Autodesk Inventor part; units mm, degrees
ref_plane "YZ Plane" through (0, 0, 0) normal (1, 0, 0) x (0, 1, 0)
ref_plane "XZ Plane" through (0, 0, 0) normal (0, 1, 0) x (-1, 0, 0)
ref_plane "XY Plane" through (0, 0, 0) normal (0, 0, 1) x (1, 0, 0)
sketch "Sketch1" plane through (0, 0, 0) normal (0, 0, 1) x (1, 0, 0)
  circle A0 centre (15.5, -7) radius 1.6
  circle A1 centre (7.75, -20.4234) radius 1.6
  circle A2 centre (-7.75, -20.4234) radius 1.6
  circle A3 centre (-15.5, -7) radius 1.6
  circle A4 centre (7.75, 6.4234) radius 1.6
  circle A5 centre (-7.75, 6.4234) radius 1.6
  circle A6 centre (0, 0) radius 6
  arc A7 (20, -7) -> (-20, -7) centre (0, -7) ccw
  line L0 (20, -7) -> (20, -32)
  line L1 (20, -32) -> (-20, -32)
  line L2 (-20, -32) -> (-20, -7)
  dimension "d0" = 40
  dimension "d1" = 25
extrude "Extrusion1" add sketch "Sketch1" along normal blind 3
sketch "Sketch2" plane through (-20, -32, 0) normal (0, -1, 0) x (1, 0, 0)
  line L0 (0, 0) -> (0, 3)
  line L1 (0, 3) -> (40, 3)
  line L2 (40, 3) -> (40, -70)
  line L3 (40, -70) -> (0, -70)
  line L4 (0, -70) -> (0, 3)
  line L5 (0, -70) -> (40, -70)
  line L6 (40, -70) -> (40, -25)
  line L7 (40, -25) -> (0, -25) construction
  line L8 (0, -25) -> (0, -70)
  line L9 (40, -25) -> (0, -70) construction
  line L10 (36.5, -30) -> (3.5, -30) construction
  line L11 (3.5, -30) -> (3.5, -65) construction
  line L12 (3.5, -65) -> (36.5, -65) construction
  line L13 (36.5, -65) -> (36.5, -30) construction
  line L14 (36.5, -30) -> (3.5, -65) construction
  line L15 (3.5, -30) -> (36.5, -65) construction
  circle A0 centre (36.5, -30) radius 1.55
  circle A1 centre (36.5, -65) radius 1.55
  circle A2 centre (3.5, -30) radius 1.55
  circle A3 centre (3.5, -65) radius 1.55
  point P0 (20, 0)
  point P1 (20, -47.5)
  dimension "d4" = 73
  dimension "d5" = 45
  dimension "d6" = 33
  dimension "d7" = 35
  dimension "d8" = 3.1
  dimension "d11" = 35
  dimension "d14" = 33
extrude "Extrusion2" add sketch "Sketch2" against normal blind 3
properties part number "Push_motor_fix"
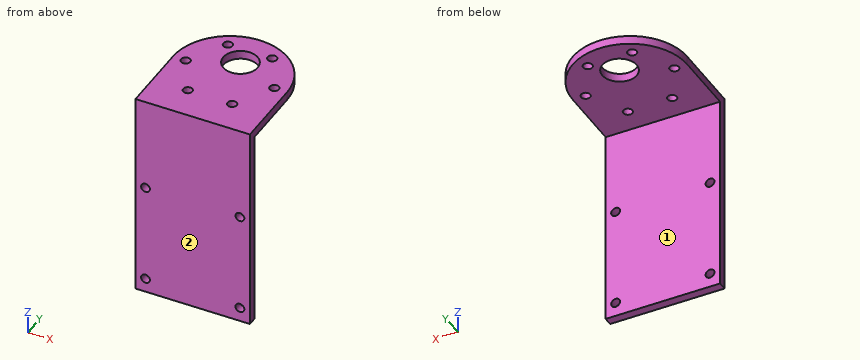
Input: part model. Units: mm. Frame: model coordinates. Face numbers are marked on the shaded views. A direction names the side the tool comes from. Coordinates: 2 decimals unless noted, no trailing zeros. Loops run counter-clockwise (first coordinate to the right, second up) from the corner with the lowest first, then second, coordinate; pieces in that order, holes last. Notation, with made-up numbers: (41, 39) -> (70, 39) arc R18 ccw to (70, 48) -> close; hole circle Ø3 at (-40, 25). An arc over 180 degrees is marked (long way). One line per item, written item: value.
(1) Pin query (flat end, axial travel): pin 1 Ø20 at (x, z) = (5, -20) entering from +Y; pin 2 Ø4 at (x, y) = (-15.5, -7) entering from -Z. Return the tip coordinate at first contact, or that it passes through.
Answer below:
pin 1: stops at y = -29
pin 2: stops at z = 0
(2) Cut plane D-D (x = -7.75). Output: boundary loops of the cut face in (y, z).
Answer below:
outline: (-32, -70) -> (-29, -70) -> (-29, 0) -> (-22.02, 0) -> (-22.02, 3) -> (-32, 3) -> close; (-18.82, 0) -> (4.82, 0) -> (4.82, 3) -> (-18.82, 3) -> close; (8.02, 0) -> (11.44, 0) -> (11.44, 3) -> (8.02, 3) -> close
(3) Set-up query: the marked faces 1 and 2. Return all of +Z, -Z, +X, -X, +Y, -Y with unobstructed straight access to the full face (end or side cutting, diameter ignored); none if empty.
Answer below:
face 1: -Z, +X, -X, +Y
face 2: +Z, -Z, +X, -X, -Y
(4) Ray query, line 1 along Z through (x, y) = (-16.5, -31.3); line 2 along Y through (x, z) = (-7, 2) (3 decimals); line 3 along Y through (x, z) = (-7.75, 2.15). Return the intervals inside material, ascending.
Answer below:
line 1: z = -70 to -66.55, -63.45 to -31.55, -28.45 to 3
line 2: y = -32 to -21.837, -19.01 to 5.01, 7.837 to 11.735
line 3: y = -32 to -22.02, -18.82 to 4.82, 8.02 to 11.44
(5) Cut plane C-C (y = -4). Output: boundary loops of the cut face in (x, z), then the cut area to 3 significant figures.
Answer below:
outline: (-19.77, 0) -> (-4.47, 0) -> (-4.47, 3) -> (-19.77, 3) -> close; (4.47, 0) -> (19.77, 0) -> (19.77, 3) -> (4.47, 3) -> close
area: 91.8 mm2
(6) Cut plane A-A (z = -30). Output: boundary loops of the cut face in (x, y), then the cut area to 3 significant figures.
Answer below:
outline: (-20, -32) -> (-18.05, -32) -> (-18.05, -29) -> (-20, -29) -> close; (-14.95, -32) -> (14.95, -32) -> (14.95, -29) -> (-14.95, -29) -> close; (18.05, -32) -> (20, -32) -> (20, -29) -> (18.05, -29) -> close
area: 101 mm2
(7) Cut plane B-B (x = -2). Output: boundary loops of the cut face in (y, z), then the cut area to 3 significant figures.
Answer below:
outline: (-32, -70) -> (-29, -70) -> (-29, 0) -> (-5.66, 0) -> (-5.66, 3) -> (-32, 3) -> close; (5.66, 0) -> (12.9, 0) -> (12.9, 3) -> (5.66, 3) -> close
area: 311 mm2
